from build123d import *

# Parameters (mm, degrees)
F0_R      = 10
F0_R_2    = 7.2
F0_R_3    = 2.7
F1_DEPTH  = 4.3
F2_DEPTH  = 0.8
F3_DEPTH  = 1
F4_R      = 4.25
F5_DEPTH  = 1
F4_W      = 10
F4_H      = 3
F6_DEPTH  = 12
F8_R      = 4.99999
F7_R      = 1.9
F9_DEPTH  = 25
F10_R     = 2
F11_DEPTH = 2.6
F12_D     = 2


# Not quite as in the source:
# - a fillet or chamfer is up to 0.001 mm smaller than in the source, because OpenCascade refuses the exact size


with BuildPart() as f1:
    # F0 (on Top) → F1 (new body)
    with BuildSketch(Plane.XY):
        with BuildLine():
            Line((0, 12.5), (-45, 12.5))
            ThreePointArc((-45, 12.5), (-52.0710678119, 9.5710678119), (-55, 2.5))
            Line((-55, 2.5), (-55, -2.5))
            ThreePointArc((-55, -2.5), (-52.0710678119, -9.5710678119), (-45, -12.5))
            Line((-45, -12.5), (0, -12.5))
            Line((0, -12.5), (0, 12.5))
        make_face()
        with Locations((-37, 0)):
            Circle(F0_R, mode=Mode.SUBTRACT)
        with Locations((-37, 0)):
            Circle(F0_R)
        with Locations((-37, 0)):
            Circle(F0_R_2, mode=Mode.SUBTRACT)
        with Locations((-37, 0)):
            Circle(F0_R_2)
        with Locations((-37, 0)):
            Circle(F0_R_3, mode=Mode.SUBTRACT)
        with Locations((-37, 0)):
            Circle(F0_R_3)
    extrude(amount=-F1_DEPTH)

    # F0 (on Top) → F2 (cut)
    with BuildSketch(Plane.XY):
        with Locations((-37, 0)):
            Circle(F0_R)
        with Locations((-37, 0)):
            Circle(F0_R_2, mode=Mode.SUBTRACT)
        with Locations((-37, 0)):
            Circle(F0_R_2)
        with Locations((-37, 0)):
            Circle(F0_R_3, mode=Mode.SUBTRACT)
    extrude(amount=-F2_DEPTH, mode=Mode.SUBTRACT)

    # F0 (on Top) → F3 (cut)
    with BuildSketch(Plane.XY):
        with Locations((-37, 0)):
            Circle(F0_R_2)
        with Locations((-37, 0)):
            Circle(F0_R_3, mode=Mode.SUBTRACT)
    extrude(amount=-F3_DEPTH, mode=Mode.SUBTRACT)

    # F4 (on face) → F5 (cut)
    with BuildSketch(Plane(origin=(0, 0, -4.3), x_dir=(1, 0, 0), z_dir=(0, 0, -1))):
        with Locations((-37, 0)):
            Circle(F4_R)
    extrude(amount=-F5_DEPTH, mode=Mode.SUBTRACT)

    # F4 (on face) → F6 (join)
    with BuildSketch(Plane(origin=(0, 0, -4.3), x_dir=(1, 0, 0), z_dir=(0, 0, -1))):
        with Locations((-5, 7)):
            Rectangle(F4_W, F4_H)
        with Locations((-5, -7)):
            Rectangle(F4_W, F4_H)
    extrude(amount=F6_DEPTH)

    # F8 (radius 5 in the source; OpenCascade refuses exactly that, so slightly less here)
    f8_edges = [f1.edges().sort_by_distance(p)[0] for p in [
        (0, -7, -16.3),
        (0, 7, -16.3),
        (-10, 7, -16.3),
        (-10, -7, -16.3),
    ]]
    fillet(f8_edges, radius=F8_R)

    # F7 (on face) → F9 (cut)
    with BuildSketch(Plane.XZ.offset(8.5)):
        with Locations((-5, -11.3)):
            Circle(F7_R)
    extrude(amount=-F9_DEPTH, mode=Mode.SUBTRACT)

    # F10
    f10_edges = [f1.edges().sort_by_distance(p)[0] for p in [
        (-22.5, -12.5, 0),
    ]]
    fillet(f10_edges, radius=F10_R)

    # F11 (cut): a face of the model
    f11_faces = [f1.faces().sort_by_distance(p)[0] for p in [
        (-37, 0, 0),
    ]]
    extrude(f11_faces, amount=-F11_DEPTH, mode=Mode.SUBTRACT)

    # F12 (through all)
    with Locations(Plane.XY):
        with Locations((-37, 0)):
            Hole(F12_D / 2)


solid = f1.part
Design review of the part built by this model. Coordinates are the model's own, in mm. A direction names the side the tool comes from. Coordinates: 2 decimals unless noted, no trailing zeros. Write each loop counter-clockwise with the first axis right and the second up, starting at its lowest first coordinate (ties: lowest second). Pieces come first, ordered by that corner, then holes. Notation, with made-up numbers: (69, 47.25) - (83, 47.25) arc R15 cw to (83, 66.25) - close; hole circle Ø11 at (-33, 46.25). An arc over 180 degrees is marked (long way). One line per item, written item: value.
1) To check wall thickness, follow probe 1 along Z at (x, y) = (-5, -6.95); probe 2 along Y at (x, z) = (-37, -3.1); probe 3 along X at (y, z) = (-7.75, -7.25). State the ranges of each line that lie inside material, in increasing order.
Answer sheet:
probe 1: z = -16.3 to -13.2, -9.4 to 0
probe 2: y = -12.5 to -1, 1 to 12.5
probe 3: x = -10 to 0
2) Add section C-C (y = 0). State the section outline as (x, z) points, plus the area to 3 significant figures.
Answer sheet:
outline: (-55, -4.3) - (-41.25, -4.3) - (-41.25, -3.3) - (-38, -3.3) - (-38, -2.6) - (-39.7, -2.6) - (-39.7, -1) - (-44.2, -1) - (-44.2, -0.8) - (-47, -0.8) - (-47, 0) - (-53, 0) arc R2 ccw to (-55, -2) - close; (-36, -3.3) - (-32.75, -3.3) - (-32.75, -4.3) - (0, -4.3) - (0, 0) - (-27, 0) - (-27, -0.8) - (-29.8, -0.8) - (-29.8, -1) - (-34.3, -1) - (-34.3, -2.6) - (-36, -2.6) - close
area: 198 mm2
3) Insertion check: pin 1 (2.5 mm diameter, centred on x = -37, y = 0, fed in from -Z); pin 2 (3 mm diameter, centred on x = -4, z = -10.5, fed in from -Y); pin 3 (10 mm diameter, centred on x = -37, y = 0, fed in from +Z). Each pin has a flat end and moves straight along its axis. Give the tip position at first contact, or say it passes through.
Answer sheet:
pin 1: stops at z = -3.3
pin 2: stops at y = -8.5
pin 3: stops at z = -1
4) Add section A-A (z = -8). State the section outline as (x, y) points, plus the area to 3 significant figures.
Answer sheet:
outline: (-10, -8.5) - (0, -8.5) - (0, -5.5) - (-10, -5.5) - close; (-10, 5.5) - (0, 5.5) - (0, 8.5) - (-10, 8.5) - close
area: 60.0 mm2
5) For faces 5 (the face through (-37, -1.2, -2.6)), 6 (the face through (-36, 1, -3.3)), 7 (the face through (-28, 0, -4.3)), 8 (the face through (-5, -8.5, -9)), 9 (the face through (-5, 5.5, -9)), list the 3-axis set-ups (+Z, -Z, +X, -X, +Y, -Y) from which the entire face can be reached by the end or side of a thin tool; tool diameter is ignored.
Answer sheet:
face 5: +Z
face 6: -Z
face 7: -Z, -X
face 8: -Z, +X, -X, -Y
face 9: -Z, +X, -X
6) Add section B-B (x = -37). State the section outline as (y, z) points.
Answer sheet:
outline: (-12.5, -4.3) - (-4.25, -4.3) - (-4.25, -3.3) - (-1, -3.3) - (-1, -2.6) - (-2.7, -2.6) - (-2.7, -1) - (-7.2, -1) - (-7.2, -0.8) - (-10, -0.8) - (-10, 0) - (-10.5, 0) arc R2 ccw to (-12.5, -2) - close; (1, -3.3) - (4.25, -3.3) - (4.25, -4.3) - (12.5, -4.3) - (12.5, -2) arc R2 ccw to (10.5, 0) - (10, 0) - (10, -0.8) - (7.2, -0.8) - (7.2, -1) - (2.7, -1) - (2.7, -2.6) - (1, -2.6) - close
7) Mouldability with a two-part tool opening along Y and no side actions: class faces 1 (the face through (-1.43, 6.98, -14.8)), 2 (the face through (-52.15, -9.49, -3.13)), 3 (the face through (-34, 0, -1)), 4 (the face through (-22, 12.5, -3)) as +Y half, -Y half, draft (parallel to the pull), parting line (faces both ways), or undercut.
Answer sheet:
face 1: draft
face 2: -Y half
face 3: undercut
face 4: +Y half
8) Add section D-D (z = -10.75). State the section outline as (x, y) points, plus the area to 3 significant figures.
Answer sheet:
outline: (-10, -8.5) - (-6.82, -8.5) - (-6.82, -5.5) - (-10, -5.5) - close; (-10, 5.5) - (-6.82, 5.5) - (-6.82, 8.5) - (-10, 8.5) - close; (-3.18, -8.5) - (0, -8.5) - (0, -5.5) - (-3.18, -5.5) - close; (-3.18, 5.5) - (0, 5.5) - (0, 8.5) - (-3.18, 8.5) - close
area: 38.2 mm2
